The figure shows three views and two pictorial views of one solid part (mm, origin at its lowest corner). Answer the questions. Round coordinates to 2 decimals unless told otherwise and drop trailing zeros. Order: outer loops, then holes, each group sorted by start corner. A loop starts at its lowest first (then second) coordinate and runs counter-clockwise, first axis right, second up. Notation, with made-up numbers: (-28.75, 36) -> (4.25, 36) arc R21 ccw to (4.25, 56) -> close; hole circle Ø5 at (68, 78). An arc over 180 degrees is marked (long way). One line per item, written item: value. Start each with the question number.
1. Section B-B (y = 12.7) is taken. Give the vertices of the cut face in (x, z) (3 decimals), then the cut area to 3 significant figures.
2. Consider line 1 (Z direction, x = 8.5, y = 10.5); line 2 (Z direction, x = 9.5, y = 14.75); line 3 (Y direction, x = 5.75, z = 25.4) (3 decimals). Determine where each line is inside the solid, lowest interval first.
3. Section A-A (z = 279.4) is taken. Give the vertices of the cut face in (x, y) (3 decimals), then the cut area to 3 significant figures.
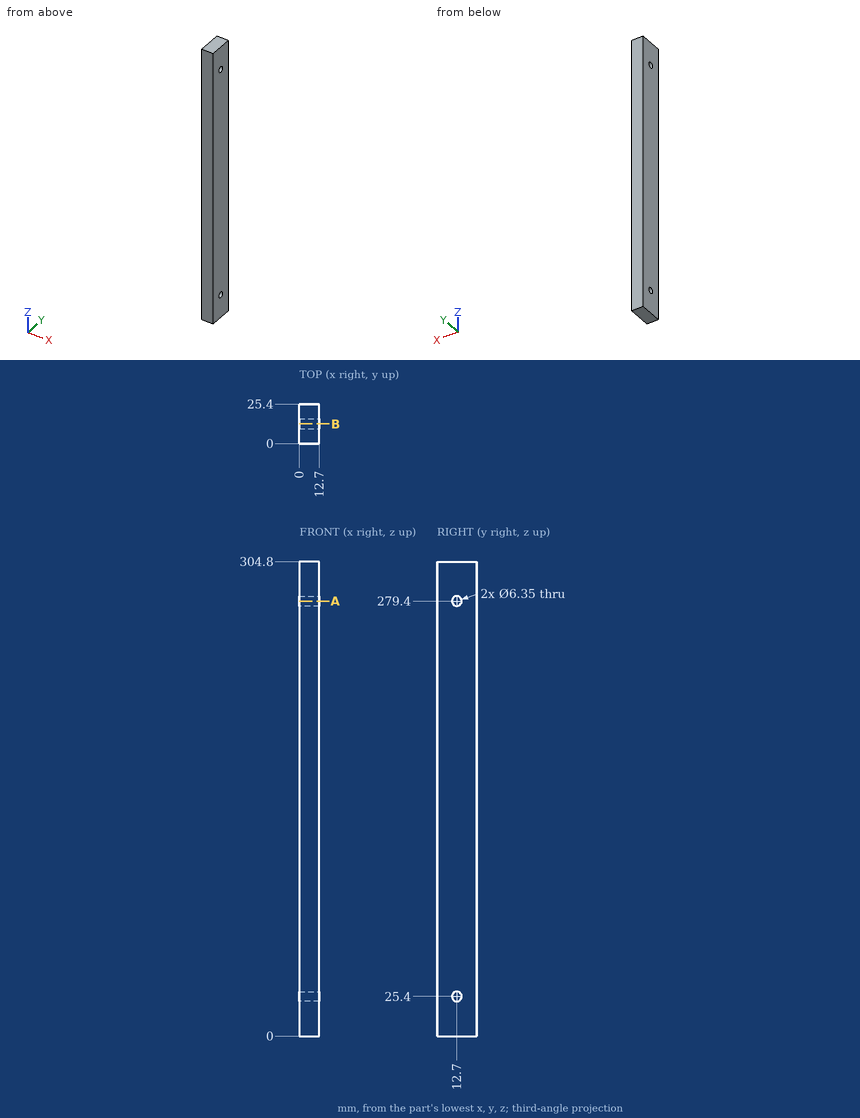
Answer:
1. outline: (0, 0) -> (12.7, 0) -> (12.7, 22.225) -> (0, 22.225) -> close; (0, 28.575) -> (12.7, 28.575) -> (12.7, 276.225) -> (0, 276.225) -> close; (0, 282.575) -> (12.7, 282.575) -> (12.7, 304.8) -> (0, 304.8) -> close
1. area: 3,710 mm^2
2. line 1: 0 to 23.11, 27.69 to 277.11, 281.69 to 304.8
2. line 2: 0 to 22.98, 27.82 to 276.98, 281.82 to 304.8
2. line 3: 0 to 9.525, 15.875 to 25.4
3. outline: (0, 0) -> (12.7, 0) -> (12.7, 9.525) -> (0, 9.525) -> close; (0, 15.875) -> (12.7, 15.875) -> (12.7, 25.4) -> (0, 25.4) -> close
3. area: 242 mm^2
